Source: three-view drawing plus pictorial views. Frame: mm from the lowest corner of the part. A direction names the side the tool comes from. Coordinates: 2 decimals unless noted, no trailing zeros. Loops run counter-clockwise (first coordinate to the right, second up) from the corner with the lowest first, then second, coordinate; pieces in that order, holes last.
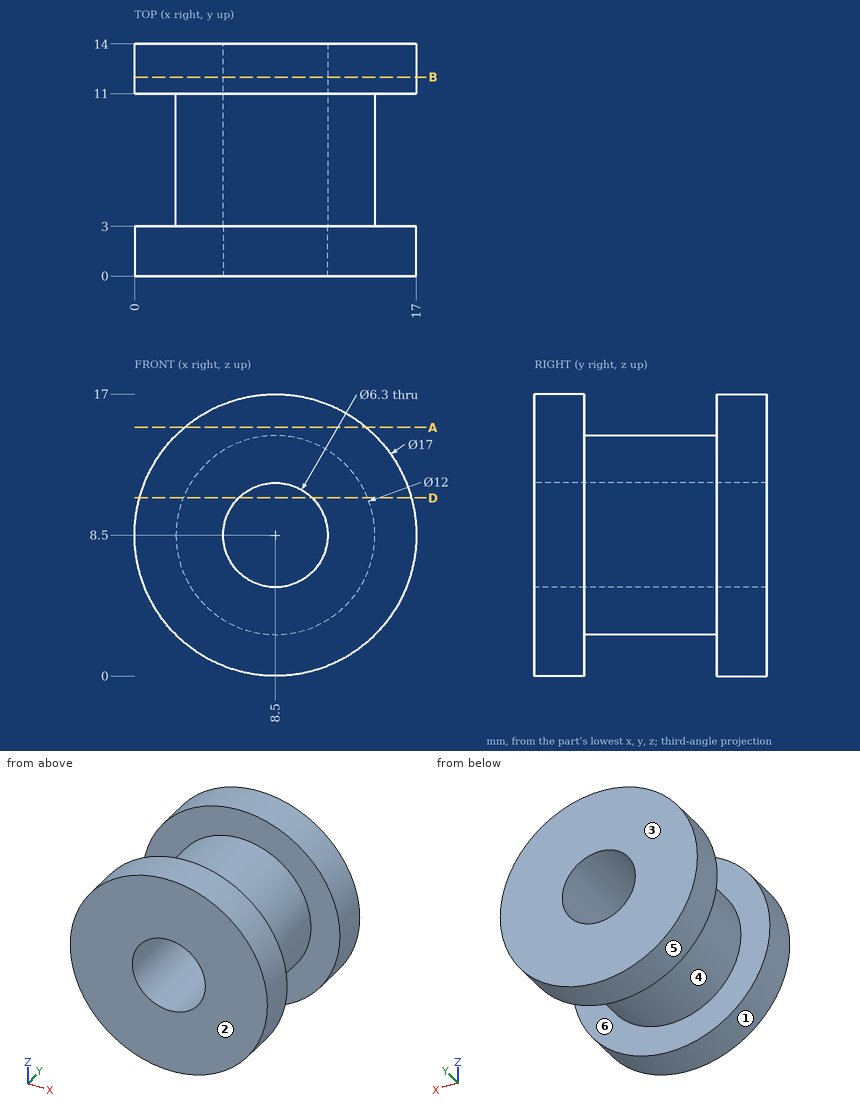
Q1. Section query B-B on y = 12. Return the cut outline in (x, z).
Q2. Draft query along Y for the marked faces 1, 2, 3 and 4. Return one class per face: released by +Y, released by -Y, zero draft, split by the parting line, or undercut.
Q3. Material intervals for line 1 along Y through (x, z) = (13, 3); line 2 along X through (y, z) = (10, 8.5), sorted ascending.
Q4. Section query D-D on z = 10.75. Return the cut outline in (x, y), then the cut area to 3 significant figures.
Q5. Section query A-A on z = 15. Return the cut outline in (x, y), then the cut area to 3 significant figures.
Q6. Reachability of the marked faces 5 and 6 from +Z, -Z, +X, -X, +Y, -Y: full face, straight path, thin tool, end or side. Return the list, or none.
Q7. First-contact query: pin 1 Ø8.5 at (x, z) = (8.5, 6.5) entering from +Y; pin 2 Ø5 at (x, y) = (6.5, 7) entering from -Z; pin 3 Ø1.5 at (x, y) = (13.5, 12) entering from +Z; pin 4 Ø4 at (x, z) = (8.5, 8.5) entering from +Y. Flat tips, straight axial feed; report the tip coordinate or a pass-through.
Resolved:
1. outline: circle Ø17 at (8.5, 8.5); hole circle Ø6.3 at (8.5, 8.5)
2. face 1: zero draft
2. face 2: released by -Y
2. face 3: released by +Y
2. face 4: undercut
3. line 1: y = 0 to 3, 11 to 14
3. line 2: x = 2.5 to 5.35, 11.65 to 14.5
4. outline: (0.3, 0) - (6.3, 0) - (6.3, 14) - (0.3, 14) - (0.3, 11) - (2.94, 11) - (2.94, 3) - (0.3, 3) - close; (10.7, 0) - (16.7, 0) - (16.7, 3) - (14.06, 3) - (14.06, 11) - (16.7, 11) - (16.7, 14) - (10.7, 14) - close
4. area: 126 mm2
5. outline: (3.02, 0) - (13.98, 0) - (13.98, 3) - (3.02, 3) - close; (3.02, 11) - (13.98, 11) - (13.98, 14) - (3.02, 14) - close
5. area: 65.7 mm2
6. face 5: +Y, -Y
6. face 6: none
7. pin 1: stops at y = 14
7. pin 2: stops at z = 2.5
7. pin 3: stops at z = 15.86
7. pin 4: passes through
